For this review, take the finished solid that the model builds, in its own axes (mm). A direction names the side the tool comes from. Give positions to 0.01 mm unless a question says otherwise; leave off trailing zeros. Order: outer loops, then holes, each group sorted by start corner. A loop starts at its lowest first (then second) coordinate and runs counter-clockwise, first axis right, second up.
from build123d import *

# Parameters (mm, degrees)
SKETCH_2_R          = 27.501856853
EXTRUDE_1_DEPTH     = 2
SKETCH_3_R          = 1.25
CUT_EXTRUDE_1_DEPTH = 2
SKETCH_4_R          = 6
CUT_EXTRUDE_2_DEPTH = 10
SKETCH_5_W          = 3
SKETCH_5_H          = 3.366075566
SKETCH_5_H_2        = 3.372140362
SKETCH_5_H_3        = 3.114077882
CUT_EXTRUDE_3_DEPTH = 10
CUT_EXTRUDE_START   = -1
CUT_EXTRUDE_4_DEPTH = 1
FILLET_1_R          = 1


with BuildPart() as part:
    # 草图2 → 凸台-拉伸1 (new body)
    with BuildSketch(Plane.XY):
        Circle(SKETCH_2_R)
    extrude(amount=EXTRUDE_1_DEPTH)

    # 草图3 → 切除-拉伸1 (cut)
    with BuildSketch(Plane.XY.offset(2)):
        with Locations((2.49431801, 19.749253685)):
            Circle(SKETCH_3_R)
        with Locations((-19.226781008, -1.971845333)):
            Circle(SKETCH_3_R)
        with Locations((2.49431801, -23.692944351)):
            Circle(SKETCH_3_R)
        with Locations((24.215417028, -1.971845333)):
            Circle(SKETCH_3_R)
    extrude(amount=-CUT_EXTRUDE_1_DEPTH, mode=Mode.SUBTRACT)

    # 草图4 → 切除-拉伸2 (cut)
    with BuildSketch(Plane.XY.offset(2)):
        with Locations((-7.485828256, 7.959275259)):
            Circle(SKETCH_4_R)
        with Locations((12.514171744, 7.959275259)):
            Circle(SKETCH_4_R)
        with Locations((-7.485828256, -12.040724741)):
            Circle(SKETCH_4_R)
        with Locations((12.514171744, -12.040724741)):
            Circle(SKETCH_4_R)
    extrude(amount=-CUT_EXTRUDE_2_DEPTH, mode=Mode.SUBTRACT)

    # 草图5 → 切除-拉伸3 (cut)
    with BuildSketch(Plane.XY.offset(2)):
        with Locations((-7.485828256, 19.276237476)):
            Rectangle(SKETCH_5_W, SKETCH_5_H)
        with Locations((12.55261862, 19.273205078)):
            Rectangle(SKETCH_5_W, SKETCH_5_H_2)
        with Locations((-7.485828256, -23.357686958)):
            Rectangle(SKETCH_5_W, SKETCH_5_H)
        with Locations((12.55261862, -23.237595759)):
            Rectangle(SKETCH_5_W, SKETCH_5_H_3)
    extrude(amount=-CUT_EXTRUDE_3_DEPTH, mode=Mode.SUBTRACT)

    # 草图6 → 切除-拉伸4 (cut)
    with BuildSketch(Plane.XY.offset(2).offset(CUT_EXTRUDE_START)):
        with BuildLine():
            Line((14.05261862, -21.680556818), (-8.985828256, -21.680556818))
            add(Edge.make_bspline(
                [(-8.985828256, -21.680556818), (-16.825868564, -20.675103315), (-22.765275429, -15.430306704)],
                knots=[0, 0, 0, 1, 1, 1], degree=2))
            ThreePointArc((-22.765275429, -15.430306704), (-24.106708477, -13.237021446), (-25.237467212, -10.928054679))
            add(Edge.make_bspline(
                [(-8.985828256, -19.180556818), (-18.318618244, -17.354029051), (-25.237467212, -10.928054679)],
                knots=[0, 0, 0, 1, 1, 1], degree=2))
            Line((-8.985828256, -19.180556818), (14.05261862, -19.180556818))
            Line((14.05261862, -19.180556818), (14.05261862, -21.680556818))
        make_face()
        with BuildLine():
            Line((14.05261862, 17.593199693), (-8.985828256, 17.593199693))
            add(Edge.make_bspline(
                [(-8.985828256, 17.593199693), (-18.141159964, 17.936782553), (-24.69378833, 12.10656633)],
                knots=[0, 0, 0, 1, 1, 1], degree=2))
            ThreePointArc((-24.69378833, 12.10656633), (-25.574531677, 10.114121805), (-26.294813962, 8.058218729))
            add(Edge.make_bspline(
                [(-8.985828256, 15.093199693), (-19.306553581, 15.286867634), (-26.294813962, 8.058218729)],
                knots=[0, 0, 0, 1, 1, 1], degree=2))
            Line((-8.985828256, 15.093199693), (14.05261862, 15.093199693))
            Line((14.05261862, 15.093199693), (14.05261862, 17.593199693))
        make_face()
    extrude(amount=CUT_EXTRUDE_4_DEPTH, mode=Mode.SUBTRACT)

    # 圆角1
    # the kernel refuses this fillet: 1 mm, written as the material it takes off along each edge
    with BuildSketch(Plane(origin=(-8.985828256, -21.674649175, 1), x_dir=(0, 0, -1), z_dir=(1, 0, 0)), Plane(origin=(-5.985828256, 17.593199693, 1), x_dir=(0, 0, -1), z_dir=(-1, 0, 0))) as fillet_1_piece_1:
        with BuildLine():
            CenterArc((FILLET_1_R, FILLET_1_R), FILLET_1_R, 180, 90)
            Line((0, FILLET_1_R), (0, 0))
            Line((0, 0), (FILLET_1_R, 0))
        make_face()
    extrude(amount=3, mode=Mode.SUBTRACT)
    with BuildSketch(Plane(origin=(14.05261862, -21.680556818, 1), x_dir=(0, 0, -1), z_dir=(-1, 0, 0)), Plane(origin=(11.05261862, 17.587134897, 1), x_dir=(0, 0, -1), z_dir=(1, 0, 0))) as fillet_1_piece_2:
        with BuildLine():
            CenterArc((FILLET_1_R, -FILLET_1_R), FILLET_1_R, 90, 90)
            Line((0, -FILLET_1_R), (0, 0))
            Line((0, 0), (FILLET_1_R, 0))
        make_face()
    extrude(amount=3, mode=Mode.SUBTRACT)


solid = part.part
1) Clearance check with flat-ended pins moving along their axes: pin 1 (0.6 mm diameter, centred on x = 12.5, z = 1, fed in from -Y); pin 2 (9.5 mm diameter, centred on x = -7.49, y = 7.96, fed in from -Z); pin 3 (5 mm diameter, centred on x = -6.5, y = -2, fed in from -Z); pin 4 (0.6 mm diameter, centred on x = -8, z = 0.5, fed in from +Y). State where each tip first meets the part, or that it passes through.
Answer sheet:
pin 1: stops at y = -21.39
pin 2: passes through
pin 3: stops at z = 0
pin 4: stops at y = 26.4
2) Draft analysis for pull direction Y (two halves, no side actions). For faces 4 (the face through (0, 2, 2)), 5 (the face through (2.223, -24.913, 1.014)), 6 (the face through (27.473, -1.25, 0.986)), state which applies: +Y half, -Y half, draft (parallel to the pull), parting line (faces both ways), or undercut.
Answer sheet:
face 4: draft
face 5: undercut
face 6: parting line
3) We need section B-B on x = -7. Give the boundary of the cut face in (y, z), then the cut area to 3 significant figures.
Answer sheet:
outline: (-26.6, 0) - (-25.04, 0) - (-25.04, 2) - (-26.6, 2) - close; (-21.67, 0) - (-18.02, 0) - (-18.02, 2) - (-19.18, 2) - (-19.18, 1) - (-20.67, 1) arc R1 ccw to start; (-6.06, 0) - (1.98, 0) - (1.98, 2) - (-6.06, 2) - close; (13.94, 0) - (17.59, 0) arc R1 ccw to (16.59, 1) - (15.09, 1) - (15.09, 2) - (13.94, 2) - close; (20.96, 0) - (26.6, 0) - (26.6, 2) - (20.96, 2) - close
area: 39.7 mm2
4) We need section A-A on x = 0. Give the boundary of the cut face in (y, z), then the cut area to 3 significant figures.
Answer sheet:
outline: (-27.5, 0) - (27.5, 0) - (27.5, 2) - (17.59, 2) - (17.59, 1) - (15.09, 1) - (15.09, 2) - (-19.18, 2) - (-19.18, 1) - (-21.68, 1) - (-21.68, 2) - (-27.5, 2) - close
area: 105 mm2
5) To check wall thickness, follow line 1 (X direction, y = -2, z = 1.95); line 2 (Y direction, x = 3.5, z = 1.25); line 3 (Y direction, x = -10, z = 0.75). State the ranges of each line that lie inside material, in increasing order.
Answer sheet:
line 1: x = -27.43 to -20.48, -17.98 to 22.97, 25.47 to 27.43
line 2: y = -27.28 to -24.44, -22.95 to -21.68, -19.18 to 15.09, 17.59 to 19.01, 20.49 to 27.28
line 3: y = -25.62 to -17.49, -6.59 to 2.51, 13.41 to 25.62
6) We need section D-D on y = -7.5. Give the boundary of the cut face in (x, z), then the cut area to 3 significant figures.
Answer sheet:
outline: (-26.46, 0) - (-11.41, 0) - (-11.41, 2) - (-26.46, 2) - close; (-3.56, 0) - (8.59, 0) - (8.59, 2) - (-3.56, 2) - close; (16.44, 0) - (26.46, 0) - (26.46, 2) - (16.44, 2) - close
area: 74.5 mm2
7) Tool access review of faces 1 (the face through (13, 20.959, 1)), 2 (the face through (14.053, -22, 1)), 3 (the face through (-5.5, -19.5, 1)): name each direction out of +Z, -Z, +X, -X, +Y, -Y from which nothing blocks a thin tool from reaching the whole face with its end or side.
Answer sheet:
face 1: +Z, -Z
face 2: +Z, -Y
face 3: +Z
8) We need section C-C on z = 0.55. Count the separate pieces of the cut face and the enclosed holes in it, then the cut area to 3 significant figures.
Answer sheet:
separate pieces: 1
enclosed holes: 11
area: 1,860 mm2
